For this review, take the finished solid that the model builds, in its own axes (mm). A direction names the side the tool comes from. Give positions to 0.01 mm unless a question says otherwise; leave off trailing zeros. Loops run counter-clockwise (first coordinate to the right, second up) from the corner with the lowest first, then second, coordinate; pieces in that order, holes last. Notation, with made-up numbers: (71.5, 6.25) - (96.5, 6.25) arc R7 ccw to (96.5, 12.25) - close; hole circle Ø4 at (77.25, -35). An arc over 180 degrees is marked (long way). Use CSV: the item, a comma, the result in double quotes. Start each with the question number.
1. Take a section at C-C on y = -14. Give the boundary of the cut face in (x, z), plus the area to 3 significant figures.
2. For pin 1 (6 mm diameter, centred on x = 11, y = 0.5, fed in from +Z); pin 2 (8 mm diameter, centred on x = 16, z = 22, fed in from +Y); pin 3 (2 mm diameter, centred on x = 17.5, z = 22.5, fed in from +Y), all flat-tipped, find the tip position at first contact; note any pin that passes through.
3. For faces 1 (the cylindrical face through (2, -14, 28)), 2 (the flat face through (10, 1, 19)), list the 3-axis set-ups (+Z, -Z, +X, -X, +Y, -Y) from which the entire face can be reached by the end or side of a thin tool; tool diameter is ignored.
4. Take a section at A-A on z = 22.5. Give the boundary of the cut face in (x, y), plus the area to 3 significant figures.
5. Wall thickness on line 1 (Z direction, x = 18, y = 9); line 2 (Y direction, x = 12, z = 17.25); line 3 (Z direction, x = 12, y = -12): over which ranges is each line inside the solid? List them lowest first.
6. Take a section at D-D on y = 2. Give the boundary of the cut face in (x, z), plus the area to 3 significant figures.
7. Take a section at B-B on x = 6.25. Give the boundary of the cut face in (y, z), plus the area to 3 significant figures.
```python
from build123d import *

# Parameters (mm, degrees)
F1_DEPTH = 20
F2_R     = 5
F3_R     = 2


with BuildPart() as f1:
    # F0 (on Right) → F1 (new body)
    with BuildSketch(Plane.YZ):
        Polygon((-17, 29), (-17, 0), (17, 0), (17, 19), (-13, 19), (-13, 29), align=None)
    extrude(amount=F1_DEPTH)

    # F2
    f2_edges = [f1.edges().sort_by_distance(p)[0] for p in [
        (20, -15, 29),
        (0, -15, 29),
        (10, 17, 19),
        (10, 17, 0),
    ]]
    fillet(f2_edges, radius=F2_R)

    # F3
    f3_edges = [f1.edges().sort_by_distance(p)[0] for p in [
        (10, -17, 0),
        (10, -17, 29),
        (10, -13, 19),
    ]]
    fillet(f3_edges, radius=F3_R)


solid = f1.part
```
Check result:
1,outline,"(0, 0) - (20, 0) - (20, 24) arc R5 ccw to (15, 29) - (5, 29) arc R5 ccw to (0, 24) - close"
1,area,"569 mm²"
2,pin 1,"stops at z = 19"
2,pin 2,"stops at y = 15"
2,pin 3,"stops at y = -13"
3,face 1,"+Z, -X, +Y, -Y"
3,face 2,"+Z, +X, -X, +Y"
4,outline,"(0, -15) arc R2 ccw to (2, -17) - (18, -17) arc R2 ccw to (20, -15) - (20, -13) - (0, -13) - close"
4,area,"78.3 mm²"
5,line 1,"z = 0 to 19"
5,line 2,"y = -17 to 15.8"
5,line 3,"z = 0 to 19.27"
6,outline,"(0, 0) - (20, 0) - (20, 19) - (0, 19) - close"
6,area,"380 mm²"
7,outline,"(-17, 2) arc R2 ccw to (-15, 0) - (12, 0) arc R5 ccw to (17, 5) - (17, 14) arc R5 ccw to (12, 19) - (-11, 19) arc R2 cw to (-13, 21) - (-13, 29) - (-15, 29) arc R2 ccw to (-17, 27) - close"
7,area,"674 mm²"
